from build123d import *

# Parameters (mm, degrees)
BOX012_W     = 94
BOX012_H     = 94
BOX012_DEPTH = 2
FILLET013_R  = 7
BOX011_W     = 100
BOX011_H     = 100
BOX011_DEPTH = 4
FILLET012_R  = 7


with BuildPart() as top_with_fillets005:
    # Box012 → Box012 (new body)
    with BuildSketch(Plane(origin=(3, 3, 2), x_dir=(1, 0, 0), z_dir=(0, 0, 1))):
        with Locations((47, 47)):
            Rectangle(BOX012_W, BOX012_H)
    extrude(amount=BOX012_DEPTH)

    # Fillet013
    fillet013_edges = [top_with_fillets005.edges().sort_by_distance(p)[0] for p in [
        (3, 3, 3),
        (3, 97, 3),
        (97, 3, 3),
        (97, 97, 3),
    ]]
    fillet(fillet013_edges, radius=FILLET013_R)


with BuildPart() as lid:
    # Box011 → Box011 (new body)
    with BuildSketch(Plane.XY):
        with Locations((50, 50)):
            Rectangle(BOX011_W, BOX011_H)
    extrude(amount=BOX011_DEPTH)

    # Fillet012
    fillet012_edges = [lid.edges().sort_by_distance(p)[0] for p in [
        (0, 0, 2),
        (0, 100, 2),
        (100, 0, 2),
        (100, 100, 2),
    ]]
    fillet(fillet012_edges, radius=FILLET012_R)

    # Cut004: cut Top with fillets005
    add(top_with_fillets005.part, mode=Mode.SUBTRACT)


with BuildPart() as lid_1:
    # Cut004 placement: moved
    add(lid.part.moved(Location((0, -110, 0))))


solid = lid_1.part
The model under review builds one solid part; all positions refer to its coordinate system, in mm. A direction names the side the tool comes from. Give positions to 0.01 mm unless a question says otherwise; leave off trailing zeros. Order: outer loops, then holes, each group sorted by start corner. A loop starts at its lowest first (then second) coordinate and runs counter-clockwise, first axis right, second up. Notation, with made-up numbers: M -38.5,80 L -23.5,80 A13 ccw -23.5,101 Z; hole C -26.75,-39.5 d1. An arc over 180 degrees is marked long. Use one line per item in the form item = value. Start each with the question number.
Item 1: We need section A-A on x = 31. Give the boundary of the cut face in (y, z).
Item 2: To check wall thickness, follow line 1 along Y through (x, z) = (33, 3.1); line 2 along X through (y, z) = (-89.5, 2.8); line 3 along Z through (x, y) = (36, -26). State the ranges of each line that lie inside material, in increasing order. Write a range as from..to.
Item 3: Insertion check: pin 1 Ø8 at (x, y) = (37.5, -26.5) entering from +Z. The pin has a flat end and moves straight along its axis. Give the tip position at first contact, or say it passes through.
Item 4: The part is to be moulded in two halves that separate along X. For faces 1 (the cylindrical face through (5, -15.1, 3)), 2 (the flat face through (0, -61, 2)), 3 (the cylindrical face through (98, -12.1, 2)), say which applies: pulls with the +X half, pulls with the -X half, needs draft (parallel to the pull), parting line crosses it, or undercut.
Item 5: We need section B-B on y = -39.5. Give the boundary of the cut face in (x, z), plus the area to 3 significant figures.
Item 6: For faces 4 (the flat face through (49, -59, 2)), 5 (the flat face through (50, -108, 4)), list the 3-axis set-ups (+Z, -Z, +X, -X, +Y, -Y) from which the entire face can be reached by the end or side of a thin tool; tool diameter is ignored.
Completed:
q1.outline = M -110,0 L -10,0 L -10,4 L -13,4 L -13,2 L -107,2 L -107,4 L -110,4 Z
q2.line_1 = -110..-107, -13..-10
q2.line_2 = 0..3, 97..100
q2.line_3 = 0..2
q3.pin_1 = 2
q4.face_1 = undercut
q4.face_2 = pulls with the -X half
q4.face_3 = pulls with the +X half
q5.outline = M 0,0 L 100,0 L 100,4 L 97,4 L 97,2 L 3,2 L 3,4 L 0,4 Z
q5.area = 212 mm²
q6.face_4 = +Z
q6.face_5 = +Z, +X, -X, +Y, -Y
